The model under review builds one solid part; all positions refer to its coordinate system, in mm. Face numbers are marked on the shaded views. A direction names the side the tool comes from. Give positions to 0.01 mm unless a question says otherwise; leave off trailing zeros. Order: outer loops, then holes, each group sorted by start corner. A loop starts at its lowest first (then second) coordinate and runs counter-clockwise, first axis right, second up. Notation, with made-up numbers: (78, 33.25) - (114, 33.25) arc R17 ccw to (114, 41.25) - close; hole circle Ø7 at (4, 11). An arc over 180 degrees is marked (long way). Put each result on its own line as item: value.
```python
from build123d import *

# Parameters (mm, degrees)
SKETCH1_R           = 4.7625
BOSS_EXTRUDE1_DEPTH = 1.27
SKETCH1_3_W         = 1.27
SKETCH1_3_H         = 36.374198342
BOSS_EXTRUDE2_DEPTH = 19.05
CUT_EXTRUDE1_DEPTH  = 33.02


with BuildPart() as part:
    # Sketch1 → Boss-Extrude1 (new body)
    with BuildSketch(Plane(origin=(0, 0, 0), x_dir=(0, 0, -1), z_dir=(1, 0, 0))):
        with BuildLine():
            Line((11.43, 20.955), (-11.43, 20.955))
            Line((-11.43, 20.955), (-11.43, -15.419198342))
            ThreePointArc((-11.43, -15.419198342), (0, -8.255), (11.43, -15.419198342))
            Line((11.43, -15.419198342), (11.43, 20.955))
        make_face()
        with Locations((0, 8.255)):
            Circle(SKETCH1_R, mode=Mode.SUBTRACT)
    extrude(amount=BOSS_EXTRUDE1_DEPTH)

    # Sketch1<3> → Boss-Extrude2 (add)
    with BuildSketch(Plane(origin=(0, 0, 0), x_dir=(0, 0, -1), z_dir=(1, 0, 0))):
        with Locations((-12.065, 2.767900829)):
            Rectangle(SKETCH1_3_W, SKETCH1_3_H)
        with Locations((12.065, 2.767900829)):
            Rectangle(SKETCH1_3_W, SKETCH1_3_H)
    extrude(amount=BOSS_EXTRUDE2_DEPTH)

    # Sketch2 → Cut-Extrude1 (cut)
    with BuildSketch(Plane.XY.offset(12.7)):
        Polygon((1.27, 20.955), (19.05, 4.445), (19.05, 20.955), align=None)
    extrude(amount=-CUT_EXTRUDE1_DEPTH, mode=Mode.SUBTRACT)


solid = part.part
```
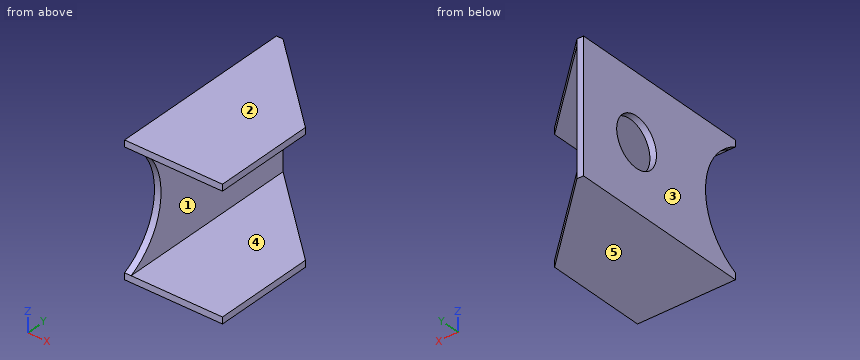
(1) The part is to be moulded in two halves that separate along Z. For the marked faces 1, 2 and 3, say which applies: pulls with the +Z half, pulls with the -Z half, needs draft (parallel to the pull), parting line crosses it, or undercut.
The answers:
face 1: undercut
face 2: pulls with the +Z half
face 3: needs draft
(2) Take a section at A-A, the plane x = 11. Write out the cut boundary in (y, z).
The answers:
outline: (-15.42, -12.7) - (11.92, -12.7) - (11.92, -11.43) - (-15.42, -11.43) - close; (-15.42, 11.43) - (11.92, 11.43) - (11.92, 12.7) - (-15.42, 12.7) - close
(3) Take a section at D-D, the plane y = -7.5. Write out the cut boundary in (x, z).
The answers:
outline: (0, -12.7) - (19.05, -12.7) - (19.05, -11.43) - (1.27, -11.43) - (1.27, 11.43) - (19.05, 11.43) - (19.05, 12.7) - (0, 12.7) - close
(4) Take a section at C-C, the plane y = 12. Write out the cut boundary in (x, z).
The answers:
outline: (0, -12.7) - (10.91, -12.7) - (10.91, -11.43) - (1.27, -11.43) - (1.27, -2.94) - (0, -2.94) - close; (0, 2.94) - (1.27, 2.94) - (1.27, 11.43) - (10.91, 11.43) - (10.91, 12.7) - (0, 12.7) - close
(5) Wall thickness on L1, parallel to Z at x = 5.75, y = -2.5; L2, parallel to Y at x = 0.8, z = 0 (1 decimal); L3, parallel to X at y = -7, z = -8.25: over which ranges is each line inside the solid? List them lowest first.
The answers:
L1: -12.7 to -11.43, 11.43 to 12.7
L2: -8.3 to 3.5, 13 to 21
L3: 0 to 1.27
(6) For the marked faces 4 and 5, list the 3-axis set-ups (+Z, -Z, +X, -X, +Y, -Y) from which the entire face can be reached by the end or side of a thin tool; tool diameter is ignored.
The answers:
face 4: +X, +Y, -Y
face 5: -Z, +X, -X, +Y, -Y
(7) Clearance check with a flat-ended pin moving along its axis: pin 1 Ø5 at (y, z) = (-6, 5.5) entering from +X. State where the tip first meets the part, or that it passes through.
The answers:
pin 1: x = 1.27
(8) Take a section at B-B, the plane z = 0. Write out the cut boundary in (x, y) (1 decimal).
The answers:
outline: (0, -8.3) - (1.3, -8.3) - (1.3, 3.5) - (0, 3.5) - close; (0, 13) - (1.3, 13) - (1.3, 21) - (0, 21) - close
